For this review, take the finished solid that the model builds, in its own axes (mm). Give positions to 0.01 mm unless a question says otherwise; leave off trailing zeros. Loops run counter-clockwise (first coordinate to the right, second up) from the corner with the lowest first, then second, coordinate; pieces in that order, holes last.
```python
from build123d import *

# Parameters (mm, degrees)
PAD_DEPTH    = 3.7
SKETCH001_W  = 0.5
SKETCH001_H  = 0.35
PAD001_DEPTH = 5


with BuildPart() as pad:
    # Sketch → Pad (new body)
    with BuildSketch(Plane.XY.offset(2.5)):
        Polygon((-0.16, 1.54), (2.7, 1.54), (3.27, 0), (3.13, -0.77), (-0.59, -0.77), (-0.73, 0), align=None)
    extrude(amount=PAD_DEPTH)


with BuildPart() as obj1:
    # Sketch001 → Pad001 (new body)
    with BuildSketch(Plane.XY.offset(2.5)):
        Rectangle(SKETCH001_W, SKETCH001_H)
        with Locations((2.54, 0)):
            Rectangle(SKETCH001_W, SKETCH001_H)
    extrude(amount=-PAD001_DEPTH)

    # obj1: union Pad
    add(pad.part)


solid = obj1.part
```
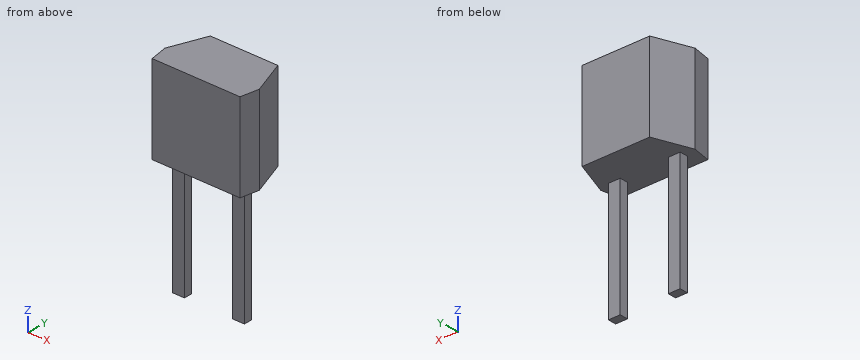
Q1. Consider section A-A on z = 0. Give the boundary of the cut face in (x, y) (3 decimals), plus the area to 3 significant figures.
Answers:
outline: (-0.25, -0.175) - (0.25, -0.175) - (0.25, 0.175) - (-0.25, 0.175) - close; (2.29, -0.175) - (2.79, -0.175) - (2.79, 0.175) - (2.29, 0.175) - close
area: 0.350 mm2
Q2. Consider section B-B on x = 0.15. Give the boundary of the cut face in (y, z) (3 decimals).
Answers:
outline: (-0.77, 2.5) - (-0.175, 2.5) - (-0.175, -2.5) - (0.175, -2.5) - (0.175, 2.5) - (1.54, 2.5) - (1.54, 6.2) - (-0.77, 6.2) - close
Q3. For probe 1 along X at (y, z) = (0.05, 1.5); probe 2 along Z at (x, y) = (2.35, 1); probe 3 along Y at (x, z) = (0.2, 1.75) (3 decimals), list the stretches that pass through material, from the lowest coordinate up.
Answers:
probe 1: x = -0.25 to 0.25, 2.29 to 2.79
probe 2: z = 2.5 to 6.2
probe 3: y = -0.175 to 0.175
Q4. For pin 1 Ø0.6 at (x, z) = (0, -1) entering from -Y (3 decimals); pin 2 Ø1 at (x, z) = (2, -1.5) entering from +Y (3 decimals), all flat-tipped, find the tip position at first contact; note any pin that passes through.
Answers:
pin 1: stops at y = -0.175
pin 2: stops at y = 0.175
Q5. Consider section C-C on z = 4.25. Give the boundary of the cut face in (x, y).
Answers:
outline: (-0.73, 0) - (-0.59, -0.77) - (3.13, -0.77) - (3.27, 0) - (2.7, 1.54) - (-0.16, 1.54) - close
Q6. Consider section D-D on y = 0.7. Give the boundary of the cut face in (x, z), plus the area to 3 significant figures.
Answers:
outline: (-0.47, 2.5) - (3.01, 2.5) - (3.01, 6.2) - (-0.47, 6.2) - close
area: 12.9 mm2
